Work out the finished part from the listing and answer in its coordinate system (mm). A direction names the side the tool comes from. Give positions to 0.01 mm unless a question says otherwise; leave off trailing zeros. Order: outer loops, then holes, each group sorted by start corner. A loop starts at its lowest first (then second) coordinate and runs counter-clockwise, first axis right, second up. Notation, with made-up numbers: (83, -21) -> (103, -21) arc R14 cw to (103, -4) -> close; hole circle Ø7 at (-7.5, 53). An arc over 180 degrees is marked (long way). Answer as CSV lines item,"result". Start each with the question number.
1. Find the intervals of material crossed by L1, parallel to Y at x = -10.75, z = 3; L2, parallel to Z at x = -2.5, y = 1.5; L3, parallel to Y at x = -1, z = 4, in increasing order.
2. For faces 5 (the flat face through (11.201, -64.389, -1.555)), 6 (the flat face through (0, -139.7, 0)), 7 (the flat face through (0, 6, 5.08)), 8 (the flat face through (0, 12.7, -6)), 9 (the cylindrical face through (-7.559, -133.261, -5.796)), determine the directions among +Z, -Z, +X, -X, +Y, -Y from which every point of the face is accessible in a straight line to the end or side of a thin tool.
3. A cutting plane is placed at A-A (x = 0). Give the vertices of the cut face in (y, z) (3 decimals), then the cut area to 3 significant figures.
4. A cutting plane is placed at C-C (y = -116). Give the vertices of the cut face in (x, z).
5. A cutting plane is placed at D-D (z = 2). Give the vertices of the cut face in (x, y), then the cut area to 3 significant figures.
6. A cutting plane is placed at B-B (z = -8). Give the vertices of the cut face in (x, y), then the cut area to 3 significant figures.
7. Flat-ended cylindrical pins translate along their axes: pin 1 (1.5 mm diameter, centred on y = -23.5, z = 7.5, fed in from -X); pin 2 (4 mm diameter, centred on x = -6, y = -10, fed in from +Z); pin 3 (5 mm diameter, centred on x = 2, y = 9.5, fed in from -Z) (3 decimals). Find the tip coordinate at first contact, or state that the pin passes through.
8. For a pull along Z with two mould halves and no side action, classify faces 1 (the flat face through (2.8, -127, -9.3)), 2 (the flat face through (5.08, 6, 0)), 3 (the flat face through (0, 0, 0)), 4 (the cylindrical face through (-12.67, -62.61, 0.86)) as released by +Z, released by -Z, zero draft, split by the parting line, or undercut.
from build123d import *

# Parameters (mm, degrees)
F0_R     = 12.7
F0_R_2   = 9.525
F0_W     = 10.16
F0_H     = 10.16
F1_DEPTH = 127
F2_DEPTH = 12.7
F3_W     = 10.16
F3_H     = 10.16
F4_DEPTH = 12.7
F5_R     = 9.525
F6_DEPTH = 12.7
F8_DEPTH = 139.701


with BuildPart() as f1:
    # F0 (on Front) → F1 (new body)
    with BuildSketch(Plane.XZ):
        Circle(F0_R)
        Circle(F0_R_2, mode=Mode.SUBTRACT)
        Circle(F0_R_2)
        Rectangle(F0_W, F0_H, mode=Mode.SUBTRACT)
        Rectangle(F0_W, F0_H)
    extrude(amount=F1_DEPTH)

    # F0 (on Front) → F2 (join)
    with BuildSketch(Plane.XZ):
        Circle(F0_R_2)
        Rectangle(F0_W, F0_H, mode=Mode.SUBTRACT)
        Rectangle(F0_W, F0_H)
    extrude(amount=-F2_DEPTH)

    # F3 (on face) → F4 (cut)
    with BuildSketch(Plane(origin=(0, 12.7, 0), x_dir=(-1, 0, 0), z_dir=(0, 1, 0))):
        Rectangle(F3_W, F3_H)
    extrude(amount=-F4_DEPTH, mode=Mode.SUBTRACT)

    # F5 (on face) → F6 (join)
    with BuildSketch(Plane.XZ.offset(127)):
        Circle(F5_R)
    extrude(amount=F6_DEPTH)

    # F7 (on face) → F8 (cut, through all)
    with BuildSketch(Plane.XZ.offset(127)):
        Polygon((14.4898414551, 1.1373524412), (12.7, 0), (9.4843178079, -2.0434010961), (9.7567712874, -2.4721587217), (14.7622949346, 0.7085948155), align=None)
    extrude(amount=-F8_DEPTH, mode=Mode.SUBTRACT)


solid = f1.part
Answer sheet:
1,L1,"y = -127 to 0"
1,L2,"z = -9.19 to -5.08, 5.08 to 9.19"
1,L3,"y = -139.7 to 0"
2,face 5,"+Y, -Y"
2,face 6,"+Z, -Z, +X, -X, -Y"
2,face 7,"+Y"
2,face 8,"+Z, -Z, +X, -X, +Y"
2,face 9,"-Y"
3,outline,"(-139.7, -9.525) -> (-127, -9.525) -> (-127, -12.7) -> (0, -12.7) -> (0, -9.525) -> (12.7, -9.525) -> (12.7, -5.08) -> (0, -5.08) -> (0, 5.08) -> (12.7, 5.08) -> (12.7, 9.525) -> (0, 9.525) -> (0, 12.7) -> (-127, 12.7) -> (-127, 9.525) -> (-139.7, 9.525) -> close"
3,area,"3,580 mm^2"
4,outline,"(9.48, -2.04) -> (12.7, 0) arc R12.7 ccw (long way) to (12.69, -0.61) -> (9.76, -2.47) -> close"
5,outline,"(-12.54, -127) -> (-9.31, -127) -> (-9.31, -139.7) -> (9.31, -139.7) -> (9.31, -127) -> (12.54, -127) -> (12.54, 0) -> (9.31, 0) -> (9.31, 12.7) -> (5.08, 12.7) -> (5.08, 0) -> (-5.08, 0) -> (-5.08, 12.7) -> (-9.31, 12.7) -> (-9.31, 0) -> (-12.54, 0) -> close"
5,area,"3,530 mm^2"
6,outline,"(-9.86, -127) -> (-5.17, -127) -> (-5.17, -139.7) -> (5.17, -139.7) -> (5.17, -127) -> (9.86, -127) -> (9.86, 0) -> (5.17, 0) -> (5.17, 12.7) -> (-5.17, 12.7) -> (-5.17, 0) -> (-9.86, 0) -> close"
6,area,"2,770 mm^2"
7,pin 1,"stops at x = -10.76"
7,pin 2,"stops at z = 12.05"
7,pin 3,"stops at z = -9.525"
8,face 1,"zero draft"
8,face 2,"undercut"
8,face 3,"undercut"
8,face 4,"split by the parting line"
